For this review, take the finished solid that the model builds, in its own axes (mm). A direction names the side the tool comes from. Give positions to 0.01 mm unless a question says otherwise; leave off trailing zeros. Loops run counter-clockwise (first coordinate to the right, second up) from the corner with the lowest first, then second, coordinate; pieces in that order, holes last. Notation, with made-up numbers: (30.25, 77.5) - (42.25, 77.5) arc R13 cw to (42.25, 86.5) - close; hole circle Ø9 at (33.5, 22). An arc over 180 degrees is marked (long way). Answer in a Markdown table with one row per item.
```python
from build123d import *

# Parameters (mm, degrees)
EXTRUDE_1_DEPTH     = 6
SKETCH_2_R          = 2
CUT_EXTRUDE_1_DEPTH = 10
SKETCH_4_R          = 1.5
CUT_EXTRUDE_2_DEPTH = 6
SKETCH_7_R          = 2
SKETCH_7_R_2        = 1.5
CUT_EXTRUDE_3_DEPTH = 6
SKETCH_5_R          = 8.5
EXTRUDE_4_DEPTH     = 5
SKETCH_14_R         = 7.55
CUT_EXTRUDE_8_DEPTH = 5
SKETCH_15_R         = 2.95
CUT_EXTRUDE_9_DEPTH = 6
FILLET_1_R          = 2


with BuildPart() as part:
    # 草图1 → 凸台-拉伸1 (new body)
    with BuildSketch(Plane(origin=(0, 0, 0), x_dir=(0, 0, -1), z_dir=(1, 0, 0))):
        Polygon((-58.108525398, 10), (-58.108525398, -35), (42.059282617, -35), (42.059282617, -30.677521513), (42.059282617, -25.387821403), (52.220185328, 2.502083897), (58.88447221, 20.794388757), (53.88447221, 20.794388757), (8.88447221, 20.794388757), (10.802160114, 26.733589605), (-8.108525398, 26.733589605), (-50.96776046, 26.733589605), align=None)
    extrude(amount=EXTRUDE_1_DEPTH)

    # 草图2 → 切除-拉伸1 (cut)
    with BuildSketch(Plane(origin=(0, 0, 0), x_dir=(0, 0, -1), z_dir=(1, 0, 0))):
        with Locations((6.512667985, -3.171691559)):
            Circle(SKETCH_2_R)
        with Locations((6.512667985, -13.171691559)):
            Circle(SKETCH_2_R)
        with Locations(Location((-42.117332015, -13.171691559, 0), (0, 0, 180))):
            Circle(SKETCH_2_R)
        with Locations(Location((-42.117332015, -3.171691559, 0), (0, 0, 180))):
            Circle(SKETCH_2_R)
        Polygon((-17.802332015, 1.828308441), (-38.302332015, 1.828308441), (-38.302332015, -18.171691559), (-17.802332015, -18.171691559), (2.697667985, -18.171691559), (2.697667985, 1.828308441), align=None)
    extrude(amount=CUT_EXTRUDE_1_DEPTH, mode=Mode.SUBTRACT)

    # 草图4 → 切除-拉伸2 (cut)
    with BuildSketch(Plane(origin=(6, 0, 0), x_dir=(0, 0, -1), z_dir=(1, 0, 0))):
        with Locations((-48.59776046, 4.328308441)):
            Circle(SKETCH_4_R)
        with Locations((48.50223954, 4.328308441)):
            Circle(SKETCH_4_R)
    extrude(amount=-CUT_EXTRUDE_2_DEPTH, mode=Mode.SUBTRACT)

    # 草图7 → 切除-拉伸3 (cut)
    with BuildSketch(Plane(origin=(6, 0, 0), x_dir=(0, 0, -1), z_dir=(1, 0, 0))):
        with Locations((-54.108525398, 6.828308441)):
            Circle(SKETCH_7_R)
        with Locations((35.891474602, -31.171691559)):
            Circle(SKETCH_7_R)
        with Locations((-54.108525398, -31.171691559)):
            Circle(SKETCH_7_R)
        with BuildLine():
            ThreePointArc((18.012667985, -3.171691559), (16.512667985, -1.671691559), (15.012667985, -3.171691559))
            Line((15.012667985, -3.171691559), (15.012667985, -23.171691559))
            ThreePointArc((15.012667985, -23.171691559), (16.512667985, -24.671691559), (18.012667985, -23.171691559))
            Line((18.012667985, -23.171691559), (18.012667985, -3.171691559))
        make_face()
        with BuildLine():
            Line((1.03223954, 18.328308441), (-47.59776046, 18.328308441))
            ThreePointArc((-47.59776046, 18.328308441), (-49.09776046, 16.828308441), (-47.59776046, 15.328308441))
            Line((-47.59776046, 15.328308441), (1.03223954, 15.328308441))
            ThreePointArc((1.03223954, 15.328308441), (2.53223954, 16.828308441), (1.03223954, 18.328308441))
        make_face()
        with BuildLine():
            Line((1.03223954, 23.328308441), (-47.59776046, 23.328308441))
            ThreePointArc((-47.59776046, 23.328308441), (-49.09776046, 21.828308441), (-47.59776046, 20.328308441))
            Line((-47.59776046, 20.328308441), (1.03223954, 20.328308441))
            ThreePointArc((1.03223954, 20.328308441), (2.53223954, 21.828308441), (1.03223954, 23.328308441))
        make_face()
        with BuildLine():
            Line((1.03223954, 13.328308441), (-47.59776046, 13.328308441))
            ThreePointArc((-47.59776046, 13.328308441), (-49.09776046, 11.828308441), (-47.59776046, 10.328308441))
            Line((-47.59776046, 10.328308441), (1.03223954, 10.328308441))
            ThreePointArc((1.03223954, 10.328308441), (2.53223954, 11.828308441), (1.03223954, 13.328308441))
        make_face()
        with BuildLine():
            ThreePointArc((38.012667985, -3.171691559), (36.512667985, -1.671691559), (35.012667985, -3.171691559))
            Line((35.012667985, -3.171691559), (35.012667985, -23.171691559))
            ThreePointArc((35.012667985, -23.171691559), (36.512667985, -24.671691559), (38.012667985, -23.171691559))
            Line((38.012667985, -23.171691559), (38.012667985, -3.171691559))
        make_face()
        with BuildLine():
            ThreePointArc((23.012667985, -3.171691559), (21.512667985, -1.671691559), (20.012667985, -3.171691559))
            Line((20.012667985, -3.171691559), (20.012667985, -23.171691559))
            ThreePointArc((20.012667985, -23.171691559), (21.512667985, -24.671691559), (23.012667985, -23.171691559))
            Line((23.012667985, -23.171691559), (23.012667985, -3.171691559))
        make_face()
        with BuildLine():
            ThreePointArc((28.012667985, -3.171691559), (26.512667985, -1.671691559), (25.012667985, -3.171691559))
            Line((25.012667985, -3.171691559), (25.012667985, -23.171691559))
            ThreePointArc((25.012667985, -23.171691559), (26.512667985, -24.671691559), (28.012667985, -23.171691559))
            Line((28.012667985, -23.171691559), (28.012667985, -3.171691559))
        make_face()
        with BuildLine():
            ThreePointArc((33.012667985, -3.171691559), (31.512667985, -1.671691559), (30.012667985, -3.171691559))
            Line((30.012667985, -3.171691559), (30.012667985, -23.171691559))
            ThreePointArc((30.012667985, -23.171691559), (31.512667985, -24.671691559), (33.012667985, -23.171691559))
            Line((33.012667985, -23.171691559), (33.012667985, -3.171691559))
        make_face()
        with Locations((-47.59776046, -28.171691559)):
            Circle(SKETCH_7_R_2)
        with Locations((29.50223954, -28.171691559)):
            Circle(SKETCH_7_R_2)
    extrude(amount=-CUT_EXTRUDE_3_DEPTH, mode=Mode.SUBTRACT)

    # 草图5 → 凸台-拉伸4 (add)
    with BuildSketch(Plane(origin=(6, 0, 0), x_dir=(0, 0, -1), z_dir=(1, 0, 0))):
        with Locations((35, 10)):
            Circle(SKETCH_5_R)
    extrude(amount=EXTRUDE_4_DEPTH)

    # 草图14 → 切除-拉伸8 (cut)
    with BuildSketch(Plane(origin=(11, 0, 0), x_dir=(0, 0, -1), z_dir=(1, 0, 0))):
        with Locations((35, 10)):
            Circle(SKETCH_14_R)
    extrude(amount=-CUT_EXTRUDE_8_DEPTH, mode=Mode.SUBTRACT)

    # 草图15 → 切除-拉伸9 (cut)
    with BuildSketch(Plane(origin=(6, 0, 0), x_dir=(0, 0, -1), z_dir=(1, 0, 0))):
        with Locations((35, 10)):
            Circle(SKETCH_15_R)
    extrude(amount=-CUT_EXTRUDE_9_DEPTH, mode=Mode.SUBTRACT)

    # 圆角1
    fillet_1_edges = [part.edges().sort_by_distance(p)[0] for p in [
        (3, 10, 58.108525398),
        (3, 26.733589605, 50.96776046),
        (3, 26.733589605, -10.802160114),
        (3, 20.794388757, -8.88447221),
        (3, 20.794388757, -58.88447221),
        (3, -25.387821403, -42.059282617),
        (3, -35, -42.059282617),
        (3, -35, 58.108525398),
    ]]
    fillet(fillet_1_edges, radius=FILLET_1_R)


solid = part.part
```
1. For faces 1 (the face through (3.042, -1.672, -31.546)), 2 (the face through (3, -11, 58.109)), 3 (the face through (8.535, 10.332, -27.457)), list the 3-axis set-ups (+Z, -Z, +X, -X, +Y, -Y) from which the entire face can be reached by the end or side of a thin tool; tool diameter is ignored.
Values:
| item | result |
|---|---|
| face 1 | +X, -X |
| face 2 | +Z, +X, -X, +Y, -Y |
| face 3 | +X |
2. We need section B-B, the plane x = 8.75. Give the boundary of the cut face in (y, z), and give its area (3 significant figures).
Values:
| item | result |
|---|---|
| outline | circle Ø17 at (10, -35); hole circle Ø15.1 at (10, -35) |
| area | 47.9 mm^2 |
3. Mouldability with a two-part tool opening along Y and no side actions: class faces 4 (the face through (3, -13, -33.013)), 5 (the face through (3, 20.794, -34)), 6 (the face through (3.04, 19.96, -57.65)) as released by +Y, released by -Y, zero draft, split by the parting line, or undercut.
Values:
| item | result |
|---|---|
| face 4 | undercut |
| face 5 | released by +Y |
| face 6 | split by the parting line |
4. We need section C-C, the plane y = -7.5. Give the boundary of the cut face in (x, z).
Values:
| item | result |
|---|---|
| outline | (0, -48.58) - (6, -48.58) - (6, -38.01) - (0, -38.01) - close; (0, -35.01) - (6, -35.01) - (6, -33.01) - (0, -33.01) - close; (0, -30.01) - (6, -30.01) - (6, -28.01) - (0, -28.01) - close; (0, -25.01) - (6, -25.01) - (6, -23.01) - (0, -23.01) - close; (0, -20.01) - (6, -20.01) - (6, -18.01) - (0, -18.01) - close; (0, -15.01) - (6, -15.01) - (6, -2.7) - (0, -2.7) - close; (0, 38.3) - (6, 38.3) - (6, 58.11) - (0, 58.11) - close |
5. We need section D-D, the plane y = 0. Give the boundary of the cut face in (x, z), and give its area (3 significant figures).
Values:
| item | result |
|---|---|
| outline | (0, -51.31) - (6, -51.31) - (6, -2.7) - (0, -2.7) - close; (0, 38.3) - (6, 38.3) - (6, 58.11) - (0, 58.11) - close |
| area | 411 mm^2 |
6. Clearance check with flat-ended pins moving along their axes: pin 1 (6.5 mm diameter, centred on x = 3.5, y = -10.5, fed in from -Z); pin 2 (5 mm diameter, centred on x = 2, y = -14, fed in from -Z); pin 3 (6 mm diameter, centred on x = 4, z = -19, fed in from +Y). State where each tip first meets the part, or that it passes through.
Values:
| item | result |
|---|---|
| pin 1 | stops at z = -48.67 |
| pin 2 | stops at z = -47.12 |
| pin 3 | stops at y = 20.79 |
7. We need section A-A, the plane z = 28. Give the boundary of the cut face in (x, y).
Values:
| item | result |
|---|---|
| outline | (0, -35) - (6, -35) - (6, -18.17) - (0, -18.17) - close; (0, 1.83) - (6, 1.83) - (6, 10.33) - (0, 10.33) - close; (0, 13.33) - (6, 13.33) - (6, 15.33) - (0, 15.33) - close; (0, 18.33) - (6, 18.33) - (6, 20.33) - (0, 20.33) - close; (0, 23.33) - (6, 23.33) - (6, 26.73) - (0, 26.73) - close |
8. Wall thickness on line 1 (Y direction, x = 4.25, z = 38); line 2 (X direction, y = -31.5, z = -7.5); line 3 (Z direction, x = 1, y = -30): over which ranges is each line inside the solid? List them lowest first. Write a range as [from, to].
Values:
| item | result |
|---|---|
| line 1 | y = [-35, -18.17], [1.83, 10.33], [13.33, 15.33], [18.33, 20.33], [23.33, 26.73] |
| line 2 | x = [0, 6] |
| line 3 | z = [-42.06, -37.51], [-34.27, 52.49], [55.73, 58.11] |
